Drawing for the job (mm, zero at the part's lowest x, y, z). A direction names the side the tool comes from. Give positions to 0.01 mm unless a question says otherwise; leave off trailing zeros. Order: outer loops, then holes, each group sorted by start corner. A loop starts at its lowest first (then second) coordinate and runs counter-clockwise, first axis right, second up. Notation, with made-up numbers: (29, 53.5) -> (76, 53.5) arc R11 cw to (76, 57.5) -> close; hole circle Ø5 at (0, 71.25). An arc over 180 degrees is marked (long way). One line per item, written item: value. Start each with the question number.
(1) Saw through at D-D on y = 13.5. Give the cut face in (x, z), plus the area to 3 significant figures.
(2) Saw through at C-C on x = 30.5. Give the cut face in (y, z).
(3) Saw through at A-A on x = 2.3. Give the cut face in (y, z).
(4) Probe line 1 (X direction, y = 17.5, z = 6); line 2 (X direction, y = 14, z = 1); line 3 (Y direction, x = 21.5, z = 5.5). List the from-to ranges inside material, lowest first.
(5) Which spindle directions (+Z, -Z, +X, -X, +Y, -Y) get a long thin tool onto all of the face, cutting with end or side? Do the marked faces 1, 2, 3 and 4. Say none if no direction does.
(6) Pin check, flat tips, straight feed: pin 1 (1.5 mm diameter, centred on x = 2, z = 7.5, fed in from +Y); pin 2 (1.5 mm diameter, centred on y = 13.5, z = 10.5, fed in from +X); pin 3 (1.5 mm diameter, centred on y = 9, z = 8.5, fed in from -X); pin 4 (8 mm diameter, centred on x = 9.5, y = 27, fed in from -Z). Stop position of each tip, or through.
(7) Saw through at B-B on z = 1.5. Give the cut face in (x, y).
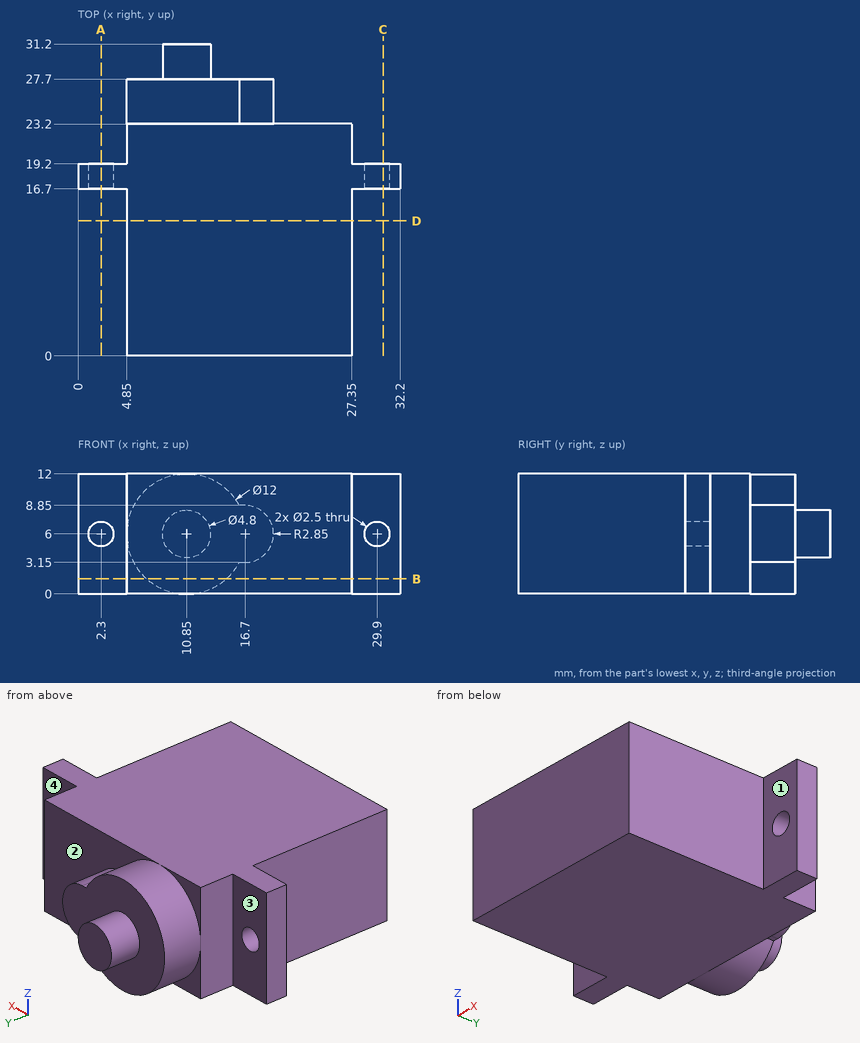
Results below:
1. outline: (4.85, 0) -> (27.35, 0) -> (27.35, 12) -> (4.85, 12) -> close
1. area: 270 mm²
2. outline: (16.7, 0) -> (19.2, 0) -> (19.2, 4.9) -> (16.7, 4.9) -> close; (16.7, 7.1) -> (19.2, 7.1) -> (19.2, 12) -> (16.7, 12) -> close
3. outline: (16.7, 0) -> (19.2, 0) -> (19.2, 4.75) -> (16.7, 4.75) -> close; (16.7, 7.25) -> (19.2, 7.25) -> (19.2, 12) -> (16.7, 12) -> close
4. line 1: x = 0 to 1.05, 3.55 to 28.65, 31.15 to 32.2
4. line 2: x = 4.85 to 27.35
4. line 3: y = 0 to 23.2
5. face 1: +Z, -Z, +X, -Y
5. face 2: +X, +Y
5. face 3: +Z, -Z, -X, +Y
5. face 4: +Z, -Z, +X, +Y
6. pin 1: stops at y = 19.2
6. pin 2: stops at x = 27.35
6. pin 3: stops at x = 4.85
6. pin 4: stops at z = 0
7. outline: (0, 16.7) -> (4.85, 16.7) -> (4.85, 0) -> (27.35, 0) -> (27.35, 16.7) -> (32.2, 16.7) -> (32.2, 19.2) -> (27.35, 19.2) -> (27.35, 23.2) -> (14.82, 23.2) -> (14.82, 27.7) -> (6.88, 27.7) -> (6.88, 23.2) -> (4.85, 23.2) -> (4.85, 19.2) -> (0, 19.2) -> close
